The drawing under review shows one solid part. Ordinate dimensions are in mm from its lowest x, y, z. A direction names the side the tool comes from. Coordinates: 2 decimals unless noted, no trailing zeros. Write each loop counter-clockwise with the first axis right and the second up, starting at its lowest first coordinate (ties: lowest second). Pieces come first, ordered by that corner, then holes.
1) Machinability: for the marked faces 5, 6 and 7, which of the approach directions +Z, -Z, +X, -X, +Y, -Y give a long, thin tool a straight path to every point of the face, cutting with its end or side? Answer none if there is none.
2) Add section A-A, the plane y = 22.5. State the section outline as (x, z) points.
3) For line 1 (Y direction, x = 12.5, z = 1.5); line 2 (X direction, y = 23, z = 0.7); line 3 (X direction, y = 16.5, z = 1), list the stretches that pass through material, from the lowest coordinate up.
4) For P1, Ø0.9, axis at x = 1.5, z = 2, coming from the -Y side; P2, Ø1.5, axis at y = 12.5, z = 2, coming from the -X side; P3, Ø5, axis at x = 3.5, y = 8.5, coming from the -Z side, all flat-tipped, find the tip position at first contact; note any pin that passes through.
5) Add section D-D, the plane x = 7. State the section outline as (y, z) points, then the cut area to 3 significant figures.
6) Add section B-B, the plane x = 12.5. State the section outline as (y, z) points, then the cut area to 3 significant figures.
7) Mouldability with a two-part tool opening along Y and no side actions: class the marked faces 1, 2, 3 and 4 as released by +Y, released by -Y, zero draft, split by the parting line, or undercut.
8) Add section C-C, the plane z = 0.6. State the section outline as (x, y) points.
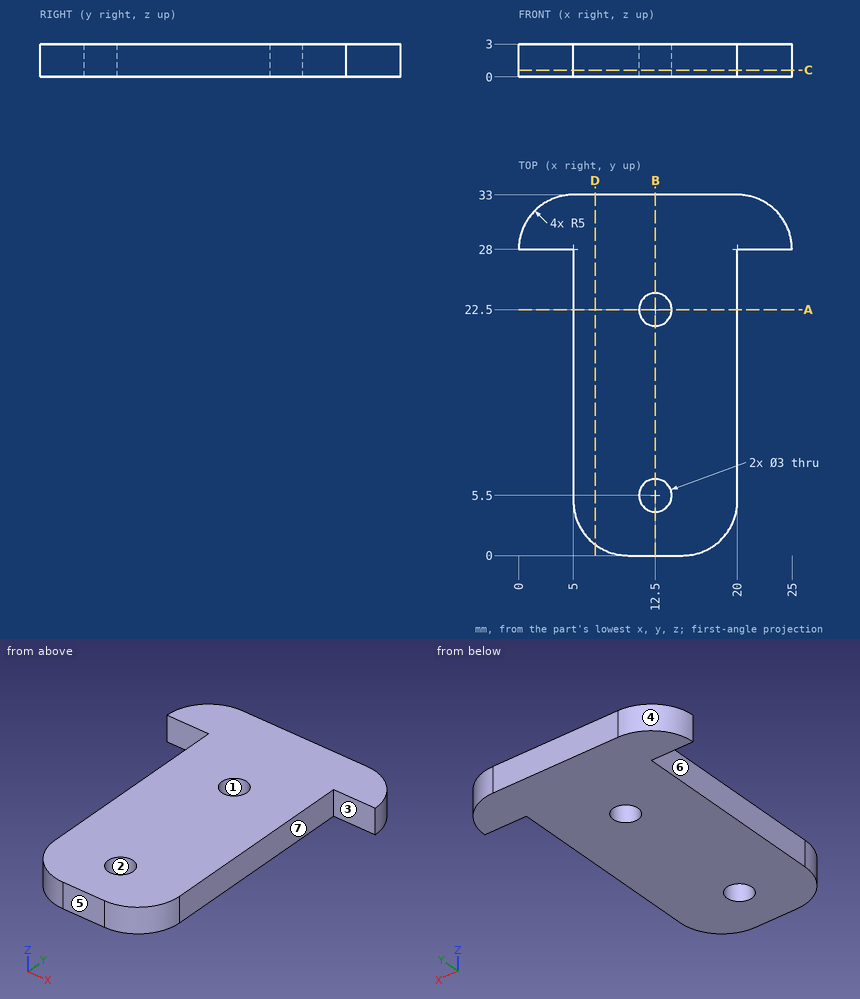
Geometry results:
1. face 5: +Z, -Z, +X, -X, -Y
1. face 6: +Z, -Z, -X, -Y
1. face 7: +Z, -Z, +X, -Y
2. outline: (5, 0) - (11, 0) - (11, 3) - (5, 3) - close; (14, 0) - (20, 0) - (20, 3) - (14, 3) - close
3. line 1: y = 0 to 4, 7 to 21, 24 to 33
3. line 2: x = 5 to 11.09, 13.91 to 20
3. line 3: x = 5 to 20
4. P1: stops at y = 28
4. P2: stops at x = 5
4. P3: stops at z = 0
5. outline: (1, 0) - (33, 0) - (33, 3) - (1, 3) - close
5. area: 96.0 mm2
6. outline: (0, 0) - (4, 0) - (4, 3) - (0, 3) - close; (7, 0) - (21, 0) - (21, 3) - (7, 3) - close; (24, 0) - (33, 0) - (33, 3) - (24, 3) - close
6. area: 81.0 mm2
7. face 1: undercut
7. face 2: undercut
7. face 3: released by -Y
7. face 4: released by +Y
8. outline: (0, 28) - (5, 28) - (5, 5) arc R5 ccw to (10, 0) - (15, 0) arc R5 ccw to (20, 5) - (20, 28) - (25, 28) arc R5 ccw to (20, 33) - (5, 33) arc R5 ccw to start; hole circle Ø3 at (12.5, 5.5); hole circle Ø3 at (12.5, 22.5)
